from build123d import *

# Parameters (mm, degrees)
F0_R     = 11.43
F1_DEPTH = 15.7734
F2_DEPTH = 40.2336
F3_R     = 3.302


with BuildPart() as f1:
    # F0 (on Top) → F1 (new body)
    with BuildSketch(Plane.XY):
        with BuildLine():
            ThreePointArc((4.8377539503, 28.162506311), (21.8491354993, 18.4159143931), (28.575, 0))
            ThreePointArc((28.575, 0), (21.8491354993, -18.4159143931), (4.8377539503, -28.162506311))
            Line((4.8377539503, -28.162506311), (59.4861693002, -18.7750042073))
            ThreePointArc((59.4861693002, -18.7750042073), (37.211, 0), (59.4861693002, 18.7750042073))
            Line((59.4861693002, 18.7750042073), (4.8377539503, 28.162506311))
        make_face()
        with BuildLine():
            ThreePointArc((75.311, 0), (70.8270903328, 12.2772762621), (59.4861693002, 18.7750042073))
            ThreePointArc((59.4861693002, 18.7750042073), (37.211, 0), (59.4861693002, -18.7750042073))
            ThreePointArc((59.4861693002, -18.7750042073), (70.8270903328, -12.2772762621), (75.311, 0))
        make_face()
        with Locations((56.261, 0)):
            Circle(F0_R, mode=Mode.SUBTRACT)
    extrude(amount=F1_DEPTH)

    # F0 (on Top) → F2 (join)
    with BuildSketch(Plane.XY):
        with BuildLine():
            ThreePointArc((4.8377539503, -28.162506311), (21.8491354993, -18.4159143931), (28.575, 0))
            ThreePointArc((28.575, 0), (21.8491354993, 18.4159143931), (4.8377539503, 28.162506311))
            ThreePointArc((4.8377539503, 28.162506311), (-28.575, 0), (4.8377539503, -28.162506311))
        make_face()
        with BuildLine():
            ThreePointArc((-13.4477648793, 4.826), (0, 14.2875), (13.4477648793, 4.826))
            Line((13.4477648793, 4.826), (18.5293, 4.826))
            Line((18.5293, 4.826), (18.5293, -4.826))
            Line((18.5293, -4.826), (13.4477648793, -4.826))
            ThreePointArc((13.4477648793, -4.826), (0, -14.2875), (-13.4477648793, -4.826))
            Line((-13.4477648793, -4.826), (-18.5293, -4.826))
            Line((-18.5293, -4.826), (-18.5293, 4.826))
            Line((-18.5293, 4.826), (-13.4477648793, 4.826))
        make_face(mode=Mode.SUBTRACT)
        with BuildLine():
            ThreePointArc((-13.4477648793, -4.826), (-14.2875, 0), (-13.4477648793, 4.826))
            Line((-13.4477648793, 4.826), (-18.5293, 4.826))
            Line((-18.5293, 4.826), (-18.5293, -4.826))
            Line((-18.5293, -4.826), (-13.4477648793, -4.826))
        make_face()
    extrude(amount=F2_DEPTH)

    # F3
    f3_edges = [f1.edges().sort_by_distance(p)[0] for p in [
        (-28.575, 0, 40.2336),
    ]]
    fillet(f3_edges, radius=F3_R)


solid = f1.part
Geometry check sheet. Reference: the model listing, model coordinates, mm. A direction names the side the tool comes from. Give positions to 0.01 mm unless a question says otherwise; leave off trailing zeros. Write each loop counter-clockwise with the first axis right and the second up, starting at its lowest first coordinate (ties: lowest second). Pieces come first, ordered by that corner, then holes. Notation, with made-up numbers: (-16.5, 69) - (18.5, 69) arc R23 ccw to (18.5, 108) - close; hole circle Ø2 at (-10.5, 41). An arc over 180 degrees is marked (long way). Put each result on its own line as item: value.
1. Go/stop test with flat-tipped pins: pin 1 (2 mm diameter, centred on y = 14, z = 12.5, fed in from -X); pin 2 (5.5 mm diameter, centred on x = 16, z = 16.5, fed in from -Y); pin 3 (12 mm diameter, centred on y = -4, z = 22, fed in from -X) (3 decimals); pin 4 (3 mm diameter, centred on y = -6, z = 29.5, fed in from -X). Record where each tip stops, or that it passes through.
Ans:
pin 1: stops at x = -25.45
pin 2: stops at y = -26.7
pin 3: stops at x = -28.575
pin 4: stops at x = -28.22
2. Sectioned sample at A-A, the plane z = 11.5. Give the number of separate pieces and of enclosed holes in the cut face, plus the area to 3 significant figures.
Ans:
separate pieces: 1
enclosed holes: 2
area: 3,480 mm²
3. Set-up check for faces 1 (the flat face through (23, 0, 0)), 2 (the cylindrical face through (-28.547, 1.256, 22.311)), 3 (the flat face through (16, -4.826, 20)): record each of +Z, -Z, +X, -X, +Y, -Y from which the full face is reachable in a straight line by a thin tool's end or side.
Ans:
face 1: -Z, +X, -X, +Y, -Y
face 2: +Z
face 3: +Z, -Z
4. Sectioned sample at D-D, the plane x = 38. Enter the section's corners in (y, z), plus the area to 3 significant figures.
Ans:
outline: (-22.47, 0) - (22.47, 0) - (22.47, 15.77) - (-22.47, 15.77) - close
area: 709 mm²
5. Thickness scan on line 1 (X direction, y = -9.5, z = 3); line 2 (X direction, y = 7.5, z = 7); line 3 (Y direction, x = 17, z = 33). Record the ranges inside material, lowest first.
Ans:
line 1: x = -26.95 to -10.67, 10.67 to 49.91, 62.62 to 72.77
line 2: x = -27.57 to -12.16, 12.16 to 47.64, 64.89 to 73.77
line 3: y = -22.97 to -4.83, 4.83 to 22.97
